For this review, use the dimensioned drawing (mm, ordinates from the lowest corner) and the shaded views. Coordinates: 2 decimals unless noted, no trailing zeros. Write each loop counter-clockwise with the first axis right and the second up, starting at its lowest first coordinate (ties: lowest second). Pieces come first, ordered by that corner, then holes. Notation, with made-up numbers: (-35.5, -15.5) - (-22.5, -15.5) arc R25 cw to (-22.5, 9.5) - close; hole circle Ø11 at (-2, -21.75). An arc over 180 degrees is marked (long way). Use one line per item in the form item = value. Start each with the question number.
1) For L1, parallel to Y at x = 8, z = 3.25 (1 decimal); L2, parallel to Y at x = 9.25, z = 8.25; L3, parallel to X at y = 26, z = 5.25 (1 decimal), list the stretches that pass through material, from the lowest coordinate up. Write a range as from..to.
2) We need section A-A (x = 7.5). Give the boundary of the cut face in (y, z) (1 decimal).
3) We need section D-D (x = 1.75). Give the boundary of the cut face in (y, z) (1 decimal), plus the area to 3 significant figures.
4) We need section B-B (y = 26). Give the boundary of the cut face in (x, z) (1 decimal).
5) Mouldability with a two-part tool opening along Y and no side actions: class the marked faces 1, 2 and 3 as pulls with the +Y half, pulls with the -Y half, needs draft (parallel to the pull), parting line crosses it, or undercut.
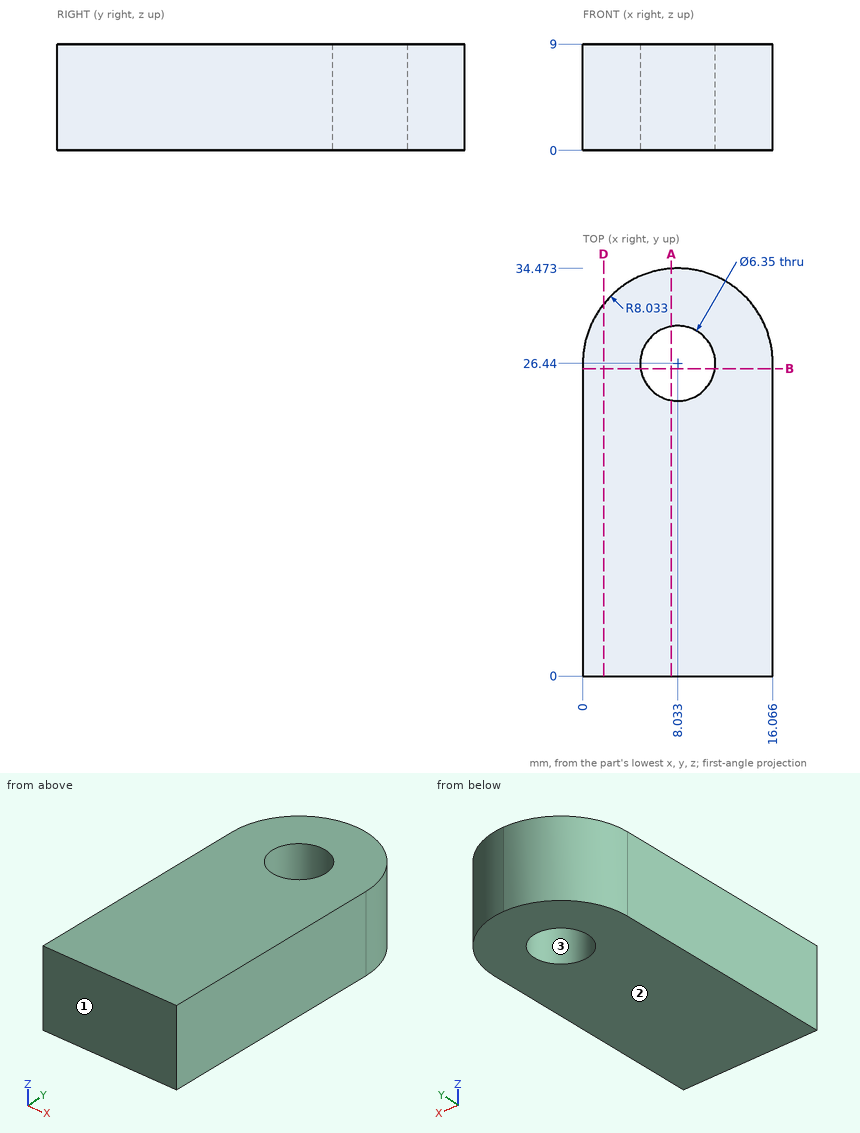
Determined:
q1.L1 = 0..23.3, 29.6..34.5
q1.L2 = 0..23.51, 29.37..34.38
q1.L3 = 0..4.9, 11.2..16.1
q2.outline = (0, 0) - (23.3, 0) - (23.3, 9) - (0, 9) - close; (29.6, 0) - (34.5, 0) - (34.5, 9) - (29.6, 9) - close
q3.outline = (0, 0) - (31.4, 0) - (31.4, 9) - (0, 9) - close
q3.area = 283 mm²
q4.outline = (0, 0) - (4.9, 0) - (4.9, 9) - (0, 9) - close; (11.2, 0) - (16.1, 0) - (16.1, 9) - (11.2, 9) - close
q5.face_1 = pulls with the -Y half
q5.face_2 = needs draft
q5.face_3 = undercut
